Read the model definition and answer for the solid it produces. Units are mm, in the model's axes. A direction names the side the tool comes from. Give positions to 0.01 mm unless a question says otherwise; leave off trailing zeros. Write each loop counter-clockwise with the first axis right and the second up, starting at its lowest first coordinate (ties: lowest second). Pieces come first, ordered by that corner, then holes. Notation, with made-up numbers: (30, -38) -> (68, -38) arc R7 cw to (68, -27) -> close; hole circle Ø8 at (-29, 65.25). An arc over 180 degrees is marked (long way). Put each result on its own line as item: value. Start each with the question number.
from build123d import *

# Parameters (mm, degrees)
F2_SIZE = 0.5


with BuildPart() as f1:
    # F0 (on Right) → F1 (revolve)
    with BuildSketch(Plane.YZ):
        Polygon((0, 7.5), (0, 4), (12, 4), (12, 7.5), (8.75, 7.5), (8.75, 7), (7.45, 7), (7.45, 7.5), align=None)
    revolve(axis=Axis((0, 6.756852, 0), (0, 1, 0)))

    # F2
    f2_edges = [f1.edges().sort_by_distance(p)[0] for p in [
        (0, 12, -7.5),
    ]]
    chamfer(f2_edges, length=F2_SIZE)

    # F3: F1 across face


with BuildPart() as f1_1:
    add(f1.part)
    add(f1.part.mirror(Plane.XZ))


solid = f1_1.part
1) Each of these flat-tipped pins is pushed along its axis until it touches: pin 1 Ø4.5 at (x, z) = (1, 3) entering from -Y; pin 2 Ø8 at (y, z) = (-5, 5) entering from +X; pin 3 Ø8 at (x, y) = (-4.5, -7) entering from +Z; pin 4 Ø1.5 at (x, y) = (-3, -4.5) entering from -Z. Where does it stop, or does it pass through?
2) Straight lines are drawn through the part: line 1 (X direction, y = 4.5, z = 0); line 2 (X direction, y = 8.5, z = 0); line 3 (Z direction, x = 1, y = -3.5). For each, find the intervals that lie inside material, in ascending order. Write a range as [from, to].
3) For faces 4 (the face through (-3, -12, -3)), 5 (the face through (2, 8.75, 7)), determine the directions among +Z, -Z, +X, -X, +Y, -Y from which every point of the face is accessible in a straight line to the end or side of a thin tool.
4) For a pull along Y with two mould halves and no side action, classify faces 1 (the face through (0.33, -10.106, -7.493)), 2 (the face through (-3, 12, -3)), 3 (the face through (2, -8.75, 7)) as pulls with the +Y half, pulls with the -Y half, needs draft (parallel to the pull), parting line crosses it, or undercut.
5) A cutting plane is placed at C-C on y = 3. Give the vertices of the cut face in (x, z), and give its area (3 significant figures).
6) A cutting plane is placed at A-A on x = 0. Give the vertices of the cut face in (y, z), and give its area (3 significant figures).
7) A cutting plane is placed at B-B on z = 0. Give the vertices of the cut face in (x, y).
Results found:
1. pin 1: stops at y = -12
1. pin 2: stops at x = 7.43
1. pin 3: stops at z = 7.48
1. pin 4: stops at z = -7.15
2. line 1: x = [-7.5, -4], [4, 7.5]
2. line 2: x = [-7, -4], [4, 7]
2. line 3: z = [-7.43, -3.87], [3.87, 7.43]
3. face 4: +Z, -Z, +X, -X, -Y
3. face 5: none
4. face 1: needs draft
4. face 2: pulls with the +Y half
4. face 3: undercut
5. outline: circle Ø15 at (0, 0); hole circle Ø8 at (0, 0)
5. area: 126 mm²
6. outline: (-12, -7) -> (-11.5, -7.5) -> (-8.75, -7.5) -> (-8.75, -7) -> (-7.45, -7) -> (-7.45, -7.5) -> (7.45, -7.5) -> (7.45, -7) -> (8.75, -7) -> (8.75, -7.5) -> (11.5, -7.5) -> (12, -7) -> (12, -4) -> (-12, -4) -> close; (-12, 4) -> (12, 4) -> (12, 7) -> (11.5, 7.5) -> (8.75, 7.5) -> (8.75, 7) -> (7.45, 7) -> (7.45, 7.5) -> (-7.45, 7.5) -> (-7.45, 7) -> (-8.75, 7) -> (-8.75, 7.5) -> (-11.5, 7.5) -> (-12, 7) -> close
6. area: 165 mm²
7. outline: (-7.5, -11.5) -> (-7, -12) -> (-4, -12) -> (-4, 12) -> (-7, 12) -> (-7.5, 11.5) -> (-7.5, 8.75) -> (-7, 8.75) -> (-7, 7.45) -> (-7.5, 7.45) -> (-7.5, -7.45) -> (-7, -7.45) -> (-7, -8.75) -> (-7.5, -8.75) -> close; (4, -12) -> (7, -12) -> (7.5, -11.5) -> (7.5, -8.75) -> (7, -8.75) -> (7, -7.45) -> (7.5, -7.45) -> (7.5, 7.45) -> (7, 7.45) -> (7, 8.75) -> (7.5, 8.75) -> (7.5, 11.5) -> (7, 12) -> (4, 12) -> close
